Source: three-view drawing plus pictorial views. Frame: mm from the lowest corner of the part. A direction names the side the tool comes from. Give positions to 0.01 mm unless a question says otherwise; leave off trailing zeros. Loops run counter-clockwise (first coordinate to the right, second up) from the corner with the lowest first, then second, coordinate; pieces in that order, holes last. Notation, with made-up numbers: (-9.75, -13.5) - (39.25, -13.5) arc R32 cw to (39.25, 25.5) - close; hole circle Ø11 at (61, -11.75). An arc over 180 degrees is marked (long way). Answer as a JSON object with one key per item and string values.
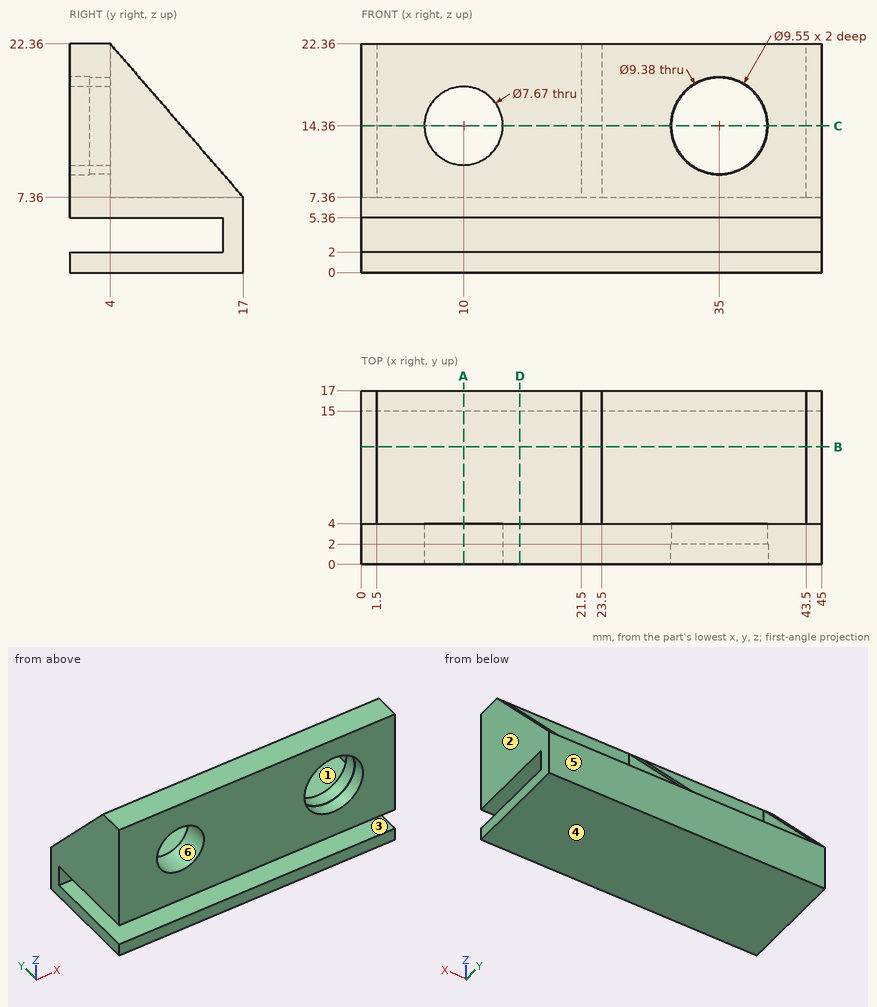
Item 1: Material intervals for line 1 (X direction, y = 14, z = 9.5); line 2 (Z direction, x = 43, y = 4.5); line 3 (Z direction, x = 31.5, y = 1.25), sorted ascending. Write a range as [from, to].
Geometry check:
{"line 1": "x = [0, 1.5], [21.5, 23.5], [43.5, 45]", "line 2": "z = [0, 2], [5.36, 7.36]", "line 3": "z = [0, 2], [5.36, 11.11], [17.61, 22.36]"}
Item 2: Cut plane C-C (z = 14.36). Return loops of the section in (x, y) (3 decimals), then the cut area to 3 significant figures.
Geometry check:
{"outline": "(0, 0) - (6.165, 0) - (6.165, 4) - (1.5, 4) - (1.5, 10.933) - (0, 10.933) - close; (13.835, 0) - (30.225, 0) - (30.225, 2) - (30.31, 2) - (30.31, 4) - (23.5, 4) - (23.5, 10.933) - (21.5, 10.933) - (21.5, 4) - (13.835, 4) - close; (39.69, 2) - (39.775, 2) - (39.775, 0) - (45, 0) - (45, 10.933) - (43.5, 10.933) - (43.5, 4) - (39.69, 4) - close", "area": "146 mm2"}
Item 3: Mould query, pull axis Z, two halves, no side actions, for the marked faces 4, 5 and 6. Classes: released by +Z, released by -Z, zero draft, split by the parting line, or undercut.
Geometry check:
{"face 4": "released by -Z", "face 5": "zero draft", "face 6": "undercut"}
Item 4: Cut plane A-A (x = 10). Return loops of the section in (y, z) (3 decimals), then the cut area to 3 significant figures.
Geometry check:
{"outline": "(0, 0) - (17, 0) - (17, 7.36) - (4, 7.36) - (4, 10.525) - (0, 10.525) - (0, 5.36) - (15, 5.36) - (15, 2) - (0, 2) - close; (0, 18.195) - (4, 18.195) - (4, 22.36) - (0, 22.36) - close", "area": "104 mm2"}
Item 5: Contact query for flat-ended pins moving along their axis: P1, Ø7.5, axis at x = 12.5, y = 9.5, coming from the +Z side; P2, Ø10, axis at x = 10, z = 14.36, coming from the +Y side. Output: stop coordinate, or through.
Geometry check:
{"P1": "stops at z = 7.36", "P2": "stops at y = 4"}
Item 6: Access query for the marked faces 1, 2 and 3. Directions: +Z, -Z, +X, -X, +Y, -Y. A direction counts if a zero-diameter tool reaches every point of the face in a straight line with its end or side. Return the directions, or none.
Geometry check:
{"face 1": "+Z, +Y", "face 2": "+Z, -Z, +X, +Y, -Y", "face 3": "+X, -X, -Y"}
Item 7: Cut plane D-D (x = 15.5). Return loops of the section in (y, z), then the cut area to 3 significant figures.
Geometry check:
{"outline": "(0, 0) - (17, 0) - (17, 7.36) - (4, 7.36) - (4, 22.36) - (0, 22.36) - (0, 5.36) - (15, 5.36) - (15, 2) - (0, 2) - close", "area": "135 mm2"}
Item 8: Cut plane B-B (y = 11.5). Return loops of the section in (x, z).
Geometry check:
{"outline": "(0, 0) - (45, 0) - (45, 2) - (0, 2) - close; (0, 5.36) - (45, 5.36) - (45, 13.71) - (43.5, 13.71) - (43.5, 7.36) - (23.5, 7.36) - (23.5, 13.71) - (21.5, 13.71) - (21.5, 7.36) - (1.5, 7.36) - (1.5, 13.71) - (0, 13.71) - close"}
